The figure shows three views and two pictorial views of one solid part (mm, origin at its lowest corner). Answer the questions. A direction names the side the tool comes from. Round coordinates to 2 decimals unless told otherwise and drop trailing zeros. Order: outer loops, then holes, each group sorted by start corner. A loop starts at its lowest first (then second) coordinate and runs counter-clockwise, first axis right, second up. Notation, with made-up numbers: (32.5, 23.25) - (65.5, 23.25) arc R16 cw to (65.5, 30.25) - close; hole circle Ø1 at (72.5, 47.5). An arc over 180 degrees is marked (long way). Answer in a Markdown table with one row per item.
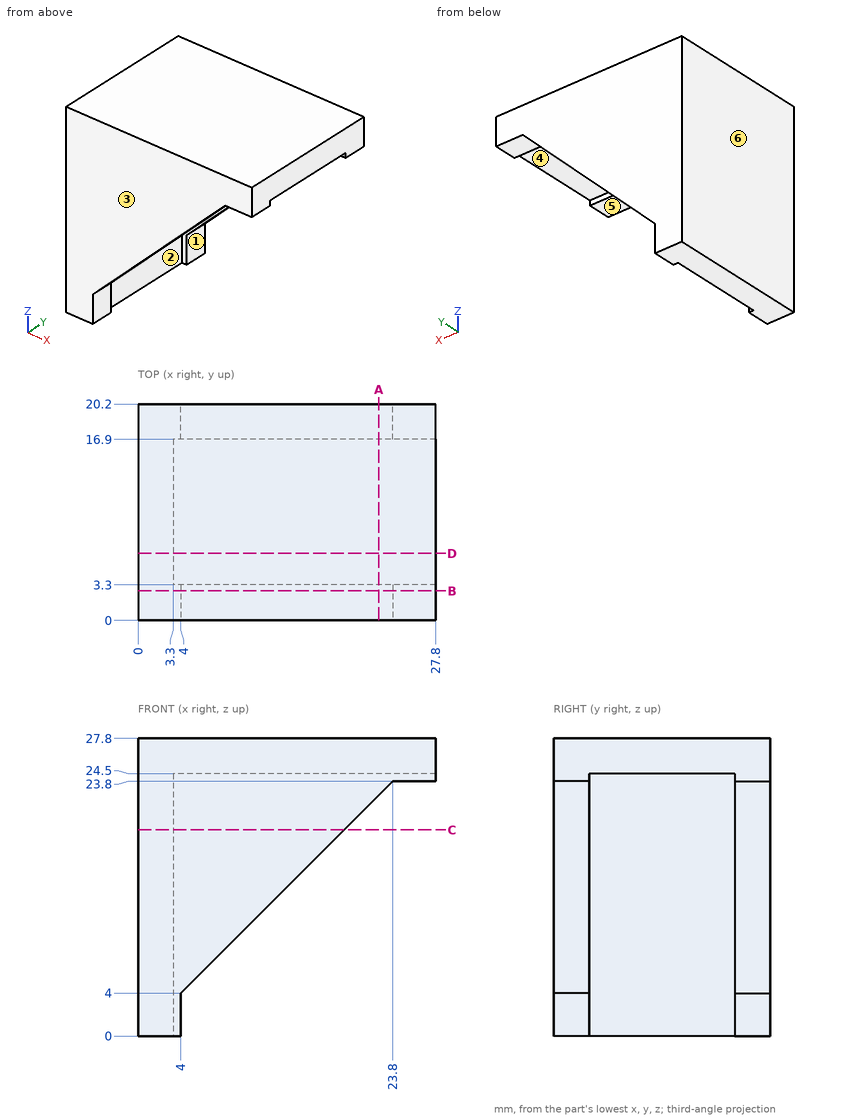
1) Find section C-C, the plane z = 19.25. Give the vertices of the cut face in (x, y).
Filled in:
| item | result |
|---|---|
| outline | (0, 0) - (19.25, 0) - (19.25, 3.3) - (3.3, 3.3) - (3.3, 16.9) - (19.25, 16.9) - (19.25, 20.2) - (0, 20.2) - close |
2) Find section A-A, the plane x = 22.5. Give the vertices of the cut face in (y, z).
Filled in:
| item | result |
|---|---|
| outline | (0, 22.5) - (3.3, 22.5) - (3.3, 24.5) - (16.9, 24.5) - (16.9, 22.5) - (20.2, 22.5) - (20.2, 27.8) - (0, 27.8) - close |
3) Find section D-D, the plane y = 6.25. Give the vertices of the cut face in (x, z), then the cut area to 3 significant figures.
Filled in:
| item | result |
|---|---|
| outline | (0, 0) - (3.3, 0) - (3.3, 24.5) - (27.8, 24.5) - (27.8, 27.8) - (0, 27.8) - close |
| area | 173 mm^2 |
4) Find the intervals of material crossed by probe 1 along Y at (x, z) = (10.25, 22); probe 2 along X at (y, z) = (13.5, 20.75); probe 3 along Z at (x, y) = (17, 5.25), in increasing order. Write a range as from..to.
Filled in:
| item | result |
|---|---|
| probe 1 | y = 0..3.3, 16.9..20.2 |
| probe 2 | x = 0..3.3 |
| probe 3 | z = 24.5..27.8 |
5) Which of the six approach directions +Z, -Z, +X, -X, +Y, -Y give full straight-line access (tool end or side, diameter ignored) to the marked faces 5 and 6?
Filled in:
| item | result |
|---|---|
| face 5 | -Z, +X, +Y, -Y |
| face 6 | +Z, -Z, -X, +Y, -Y |
6) Each of these flat-tipped pins is pushed along its axis until it touches: pin 1 (11 mm diameter, centred on x = 17.5, y = 10.5, fed in from -Z); pin 2 (2.5 mm diameter, centred on x = 26.5, y = 19, fed in from -Z); pin 3 (1.7 mm diameter, centred on y = 19, z = 2, fed in from +X). Where does it stop, or does it pass through?
Filled in:
| item | result |
|---|---|
| pin 1 | stops at z = 24.5 |
| pin 2 | stops at z = 23.8 |
| pin 3 | stops at x = 4 |
7) Find section B-B, the plane y = 2.75. Give the vertices of the cut face in (x, z).
Filled in:
| item | result |
|---|---|
| outline | (0, 0) - (4, 0) - (4, 4) - (23.8, 23.8) - (27.8, 23.8) - (27.8, 27.8) - (0, 27.8) - close |
8) The mould has two halves that part along Y. Classify the marked faces 1, 2, 3 and 4: released by +Y, released by -Y, zero draft, split by the parting line, or undercut.
Filled in:
| item | result |
|---|---|
| face 1 | zero draft |
| face 2 | undercut |
| face 3 | released by -Y |
| face 4 | undercut |
